CAD build for the part. Positions are in the model's coordinates, mm. Face numbers are marked on the shaded views. A direction names the side the tool comes from. Give positions to 0.01 mm unless a question says otherwise; leave off trailing zeros. Loops run counter-clockwise (first coordinate to the right, second up) from the corner with the lowest first, then second, coordinate; pieces in that order, holes last. Notation, with made-up numbers: (60, 82) - (82, 82) arc R26 cw to (82, 109) - close; hole circle Ø7 at (40, -25). An arc over 180 degrees is marked (long way). Return JSON: item names as keys, results as strings.
from build123d import *

# Parameters (mm, degrees)
SKETCH1_R                            = 9
SKETCH1_R_2                          = 4.45
BOSS_EXTRUDE1_DEPTH                  = 6.5
CUT_EXTRUDE1_START                   = -4.9
SKETCH2_R                            = 9
SKETCH2_R_2                          = 7.25
CUT_EXTRUDE1_DEPTH                   = 4.9
SKETCH4_R                            = 6.3
SKETCH4_R_2                          = 4.45
CUT_EXTRUDE2_DEPTH                   = 0.3
SKETCH5_R                            = 9
SKETCH5_R_2                          = 6.8
CUT_EXTRUDE3_DEPTH                   = 0.6
SKETCH6_R                            = 8.5
SKETCH6_R_2                          = 6.8
CUT_EXTRUDE4_DEPTH                   = 0.3
SKETCH7_R                            = 6.5
CUT_EXTRUDE5_DEPTH                   = 5
SKETCH8_R                            = 5.4
CUT_EXTRUDE6_DEPTH                   = 1
BOSS_EXTRUDE5_REACH                  = 21.68
BOSS_EXTRUDE5_END_RADIUS             = 9
BOSS_EXTRUDE5_DIRECTION_2_REACH      = 21.68
BOSS_EXTRUDE5_DIRECTION_2_END_RADIUS = 7.25
SKETCH11_R                           = 0.5
CUT_EXTRUDE7_DEPTH                   = 15.291606127
SKETCH12_R                           = 8
SKETCH12_R_2                         = 6.8
CUT_EXTRUDE8_DEPTH                   = 0.2


with BuildPart() as part:
    # Sketch1 → Boss-Extrude1 (new body)
    with BuildSketch(Plane.XY):
        Circle(SKETCH1_R)
        Circle(SKETCH1_R_2, mode=Mode.SUBTRACT)
    extrude(amount=-BOSS_EXTRUDE1_DEPTH)

    # Sketch2 → Cut-Extrude1 (cut)
    with BuildSketch(Plane(origin=(0, 0, -6.5), x_dir=(-1, 0, 0), z_dir=(0, 0, -1)).offset(CUT_EXTRUDE1_START)):
        with Locations(Location((0, 0, 0), (0, 0, 180))):
            Circle(SKETCH2_R)
        Circle(SKETCH2_R_2, mode=Mode.SUBTRACT)
    extrude(amount=CUT_EXTRUDE1_DEPTH, mode=Mode.SUBTRACT)

    # Sketch4 → Cut-Extrude2 (cut)
    with BuildSketch(Plane.XY):
        Circle(SKETCH4_R)
        Circle(SKETCH4_R_2, mode=Mode.SUBTRACT)
    extrude(amount=-CUT_EXTRUDE2_DEPTH, mode=Mode.SUBTRACT)

    # Sketch5 → Cut-Extrude3 (cut)
    with BuildSketch(Plane.XY):
        Circle(SKETCH5_R)
        Circle(SKETCH5_R_2, mode=Mode.SUBTRACT)
    extrude(amount=-CUT_EXTRUDE3_DEPTH, mode=Mode.SUBTRACT)

    # Sketch6 → Cut-Extrude4 (cut)
    with BuildSketch(Plane.XY.offset(-0.6)):
        Circle(SKETCH6_R)
        Circle(SKETCH6_R_2, mode=Mode.SUBTRACT)
    extrude(amount=-CUT_EXTRUDE4_DEPTH, mode=Mode.SUBTRACT)

    # Sketch7 → Cut-Extrude5 (cut)
    with BuildSketch(Plane(origin=(0, 0, -6.5), x_dir=(-1, 0, 0), z_dir=(0, 0, -1))):
        Circle(SKETCH7_R)
    extrude(amount=-CUT_EXTRUDE5_DEPTH, mode=Mode.SUBTRACT)

    # Sketch8 → Cut-Extrude6 (cut)
    with BuildSketch(Plane(origin=(0, 0, -1.5), x_dir=(-1, 0, 0), z_dir=(0, 0, -1))):
        Circle(SKETCH8_R)
    extrude(amount=-CUT_EXTRUDE6_DEPTH, mode=Mode.SUBTRACT)


with BuildPart() as body_2:
    # Boss-Extrude5: up to this cylinder (the profile starts inside it)
    boss_extrude5_end = Plane(origin=(0, 0, -3.492216), z_dir=(0, 0, 1)) * Cylinder(BOSS_EXTRUDE5_END_RADIUS, 62.36, mode=Mode.PRIVATE)
    # Sketch9 → Boss-Extrude5 (new, up to the surface)
    with BuildSketch(Plane(origin=(0, 7.25, 0), x_dir=(1, 0, 0), z_dir=(0, 1, 0)), mode=Mode.PRIVATE) as boss_extrude5_sk1:
        with BuildLine():
            Line((-1.35, 1.6), (-1.35, 4.3))
            ThreePointArc((-1.35, 4.3), (0, 5.65), (1.35, 4.3))
            Line((1.35, 4.3), (1.35, 1.6))
            Line((1.35, 1.6), (-1.35, 1.6))
        make_face()
    boss_extrude5_tool1 = extrude(boss_extrude5_sk1.sketch, amount=BOSS_EXTRUDE5_REACH, mode=Mode.PRIVATE) & boss_extrude5_end
    add(boss_extrude5_tool1.solids().sort_by_distance((0, 7.25, -3.492216))[0])

    # Boss-Extrude5 direction 2: up to this cylinder (the profile starts outside it)
    boss_extrude5_direction_2_end = Plane(origin=(0, 0, -3.492216), z_dir=(0, 0, -1)) * Cylinder(BOSS_EXTRUDE5_DIRECTION_2_END_RADIUS, 58.86, mode=Mode.PRIVATE)
    # Sketch9 → Boss-Extrude5 direction 2 (add, up to the surface)
    with BuildSketch(Plane(origin=(0, 7.25, 0), x_dir=(1, 0, 0), z_dir=(0, 1, 0)), mode=Mode.PRIVATE) as boss_extrude5_direction_2_sk1:
        with BuildLine():
            Line((-1.35, 1.6), (-1.35, 4.3))
            ThreePointArc((-1.35, 4.3), (0, 5.65), (1.35, 4.3))
            Line((1.35, 4.3), (1.35, 1.6))
            Line((1.35, 1.6), (-1.35, 1.6))
        make_face()
    boss_extrude5_direction_2_tool1 = extrude(boss_extrude5_direction_2_sk1.sketch, amount=-BOSS_EXTRUDE5_DIRECTION_2_REACH, mode=Mode.PRIVATE) - boss_extrude5_direction_2_end
    add(boss_extrude5_direction_2_tool1.solids().sort_by_distance((0, 7.25, -3.492216))[0])
    add(boss_extrude5_direction_2_tool1.solids().sort_by_distance((0, 7.25, -3.492216))[1])


with BuildPart() as body_3:
    # Mirror2: mirrored copy
    add(body_2.part.mirror(Plane.ZX))


with BuildPart() as body_2_1:
    add(body_2.part)

    # Combine3: union part, body 3
    add(part.part)
    add(body_3.part)

    # Sketch11 → Cut-Extrude7 (cut, through all)
    with BuildSketch(Plane(origin=(0, 0, 0), x_dir=(1, 0, 0), z_dir=(0, 1, 0))):
        with Locations(Location((0, 3.1, 0), (0, 0, 270))):
            Circle(SKETCH11_R)
    extrude(amount=-CUT_EXTRUDE7_DEPTH, mode=Mode.SUBTRACT)

    # Sketch12 → Cut-Extrude8 (cut)
    with BuildSketch(Plane.XY.offset(-0.9)):
        Circle(SKETCH12_R)
        Circle(SKETCH12_R_2, mode=Mode.SUBTRACT)
    extrude(amount=-CUT_EXTRUDE8_DEPTH, mode=Mode.SUBTRACT)


solid = body_2_1.part
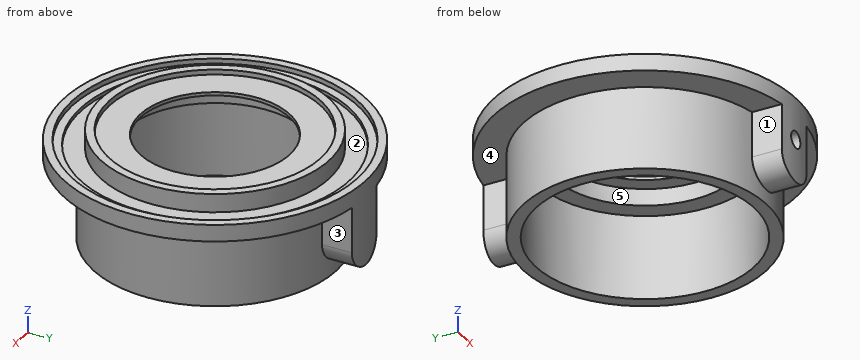
1. Cut at D-D, the plane z = -3.1. Write the cut outline in (x, y), plus the area to 3 significant figures.
Values follow:
{"outline": "(-1.35, -8.9) arc R9 ccw to (-0.5, -8.99) - (-0.5, -6.48) arc R6.5 cw (long way) to (0.5, -6.48) - (0.5, -8.99) arc R9 ccw to (1.35, -8.9) - (1.35, -7.12) arc R7.25 ccw to (1.35, 7.12) - (1.35, 8.9) arc R9 ccw to (-1.35, 8.9) - (-1.35, 7.12) arc R7.25 ccw to (-1.35, -7.12) - close", "area": "39.4 mm²"}
2. Which spindle directions (+Z, -Z, +X, -X, +Y, -Y) get a long thin tool onto all of the face, cutting with end or side? Do the marked faces 1, 2, 3, 4 and 5. Say none if no direction does.
Values follow:
{"face 1": "-Z, -X, -Y", "face 2": "+Z", "face 3": "-Z, +X, +Y", "face 4": "-Z, -X", "face 5": "-Z"}
3. Drill centre lines: probe 1 along Y at (x, z) = (0, -0.75); probe 2 along X at (y, z) = (-0.25, -1.75); probe 3 along Y at (x, z) = (4.25, -1). Where is each one in solid material? Low to high.
Values follow:
{"probe 1": "y = -9 to -8.5, -6.8 to -5.4, 5.4 to 6.8, 8.5 to 9", "probe 2": "x = -7.25 to -6.5, 6.5 to 7.25", "probe 3": "y = -7.93 to -6.78, -5.31 to -3.33, 3.33 to 5.31, 6.78 to 7.93"}
4. Cut at C-C, the plane x = 0. Give the number of separate pieces and of enclosed holes in the cut face, plus the area to 3 significant figures.
Values follow:
{"separate pieces": "3", "enclosed holes": "0", "area": "26.0 mm²"}
5. Drop flat-ended pins along their axis: P1, Ø2, axis at x = 1, z = -4.5, coming from the +Y side; P2, Ø2, axis at x = 1, y = 4.5, coming from the -Z side; P3, Ø3, axis at y = -7, z = -4, coming from the +X side; P4, Ø2, axis at x = -6.5, y = 5.5, coming from the +Z side. Give the stop position or say it passes through.
Values follow:
{"P1": "stops at y = 9", "P2": "stops at z = -1.5", "P3": "stops at x = 4.72", "P4": "stops at z = -0.6"}
6. Cut at B-B, the plane z = -5. Write the cut outline in (x, y), plus the area to 3 significant figures.
Values follow:
{"outline": "(-1.15, -8.93) arc R9 ccw to (1.15, -8.93) - (1.15, -7.16) arc R7.25 ccw to (1.15, 7.16) - (1.15, 8.93) arc R9 ccw to (-1.15, 8.93) - (-1.15, 7.16) arc R7.25 ccw to (-1.15, -7.16) - close; hole circle Ø13 at (0, 0)", "area": "40.5 mm²"}
